```python
from build123d import *

# Parameters (mm, degrees)
F0_R     = 28.575
F1_DEPTH = 64
F0_R_2   = 11.1
F2_DEPTH = 44
F3_W     = 10
F3_H     = 38
F4_DEPTH = 54
F6_W     = 22
F6_H     = 50
F7_DEPTH = 114
F9_DEPTH = 41


with BuildPart() as f1:
    # F0 (on Front) → F1 (new body)
    with BuildSketch(Plane.XZ):
        with BuildLine():
            ThreePointArc((35.1425667816, -41), (49.0596504584, -22.5643678594), (54, 0))
            ThreePointArc((54, 0), (49.0596504584, 22.5643678594), (35.1425667816, 41))
            ThreePointArc((35.1425667816, 41), (-54, 0), (35.1425667816, -41))
        make_face()
        Circle(F0_R, mode=Mode.SUBTRACT)
    extrude(amount=F1_DEPTH)

    # F0 (on Front) → F2 (join)
    with BuildSketch(Plane.XZ):
        with BuildLine():
            ThreePointArc((35.1425667816, 41), (49.0596504584, 22.5643678594), (54, 0))
            ThreePointArc((54, 0), (49.0596504584, -22.5643678594), (35.1425667816, -41))
            Line((35.1425667816, -41), (174, -41))
            Line((174, -41), (174, 41))
            Line((174, 41), (35.1425667816, 41))
        make_face()
        with Locations((89, 0)):
            Circle(F0_R_2, mode=Mode.SUBTRACT)
        with Locations((139, 0)):
            Circle(F0_R_2, mode=Mode.SUBTRACT)
    extrude(amount=F2_DEPTH)

    # F3 (on Right) → F4 (cut, symmetric)
    with BuildSketch(Plane.YZ):
        with Locations((-59, -35)):
            Rectangle(F3_W, F3_H)
        with Locations((-59, 35)):
            Rectangle(F3_W, F3_H)
    extrude(amount=F4_DEPTH, both=True, mode=Mode.SUBTRACT)

    # F6 (on offset) → F7 (cut)
    with BuildSketch(Plane.YZ.offset(174)):
        with Locations((-33, 0)):
            Rectangle(F6_W, F6_H)
    extrude(amount=-F7_DEPTH, mode=Mode.SUBTRACT)

    # F8 (on Top) → F9 (cut, symmetric)
    with BuildSketch(Plane.XY):
        Polygon((174, -32), (162, -44), (174, -44), align=None)
    extrude(amount=F9_DEPTH, both=True, mode=Mode.SUBTRACT)


solid = f1.part
```
Check sheet for the modelled part. Datum: model origin and axes. Units: mm. A direction names the side the tool comes from. Round coordinates to 2 decimals unless told otherwise and drop trailing zeros. Loops run counter-clockwise (first coordinate to the right, second up) from the corner with the lowest first, then second, coordinate; pieces in that order, holes last. Notation, with made-up numbers: (71.5, 16.5) -> (116.5, 16.5) arc R20 ccw to (116.5, 25.5) -> close; hole circle Ø2 at (84.5, 9). An arc over 180 degrees is marked (long way). Write item = value, one per line. Start each with the question number.
1) Sectioned sample at B-B, the plane y = -40. Record the cut outline in (x, z) (3 decimals), plus the area to 3 significant figures.
2) Thickness scan on probe 1 along X at (y, z) = (-41.5, 1); probe 2 along Z at (x, y) = (99, -43); probe 3 along Z at (x, y) = (139, -8.75). Record the ranges inside material, lowest first.
3) Set-up check for faces 4 (the flat face through (104, -22, -41)), 5 (the flat face through (37, -59, -16)), 6 (the flat face through (38, -59, 16)), 7 (the flat face through (106, -22, 41)), 8 (the flat face through (60, -33, 0)): record each of +Z, -Z, +X, -X, +Y, -Y from which the full face is reachable in a straight line by a thin tool's end or side.
4) Sectioned sample at C-C, the plane y = -16.5. Record the cut outline in (x, z) (3 decimals), plus the area to 3 significant figures.
5) Sectioned sample at A-A, the plane x = 139. Record the cut outline in (y, z), plus the area to 3 significant figures.
6) Gauge pin test, flat ends, axial feed: pin 1 Ø4 at (x, y) = (72.5, -45.5) entering from +Z; pin 2 Ø5 at (y, z) = (-54, -6) entering from +X; pin 3 Ø10 at (x, z) = (66, -39) entering from -Y; pin 4 Ø4 at (x, z) = (-15, -33.5) entering from +Y. Record the tip position at first contact, or that the pin passes through.
7) Release check for a two-part mould opening along Z. For faces 1 (the cylindrical face through (99.254, -10.846, -4.251)), 2 (the flat face through (-37, -59, 16)), 3 (the flat face through (168, -38, -33)) record: released by +Z, released by -Z, zero draft, split by the parting line, or undercut.
8) Sectioned sample at D-D, the plane x = 0. Record the cut outline in (y, z) (3 decimals).
Results are:
q1.outline = (35.143, -41) -> (166, -41) -> (166, -25) -> (60, -25) -> (60, 25) -> (166, 25) -> (166, 41) -> (35.143, 41) arc R54 ccw (long way) to start; hole circle Ø57.15 at (0, 0)
q1.area = 11,000 mm^2
q2.probe_1 = -53.99 to -28.56, 28.56 to 60
q2.probe_2 = -41 to -25, 25 to 41
q2.probe_3 = -41 to -11.1, 11.1 to 41
q3.face_4 = -Z, +X, +Y, -Y
q3.face_5 = -Z, +X, -X, -Y
q3.face_6 = +Z, +X, -X, -Y
q3.face_7 = +Z, +X, +Y, -Y
q3.face_8 = +X, -Y
q4.outline = (35.143, -41) -> (174, -41) -> (174, 41) -> (35.143, 41) arc R54 ccw (long way) to start; hole circle Ø57.15 at (0, 0); hole circle Ø22.2 at (89, 0); hole circle Ø22.2 at (139, 0)
q4.area = 16,100 mm^2
q5.outline = (-44, -41) -> (0, -41) -> (0, -11.1) -> (-22, -11.1) -> (-22, -25) -> (-44, -25) -> close; (-44, 25) -> (-22, 25) -> (-22, 11.1) -> (0, 11.1) -> (0, 41) -> (-44, 41) -> close
q5.area = 2,020 mm^2
q6.pin_1 = 41
q6.pin_2 = 53.89
q6.pin_3 = -44
q6.pin_4 = 0
q7.face_1 = undercut
q7.face_2 = released by +Z
q7.face_3 = zero draft
q8.outline = (-54, -54) -> (0, -54) -> (0, -28.575) -> (-54, -28.575) -> close; (-54, 28.575) -> (0, 28.575) -> (0, 54) -> (-54, 54) -> close
